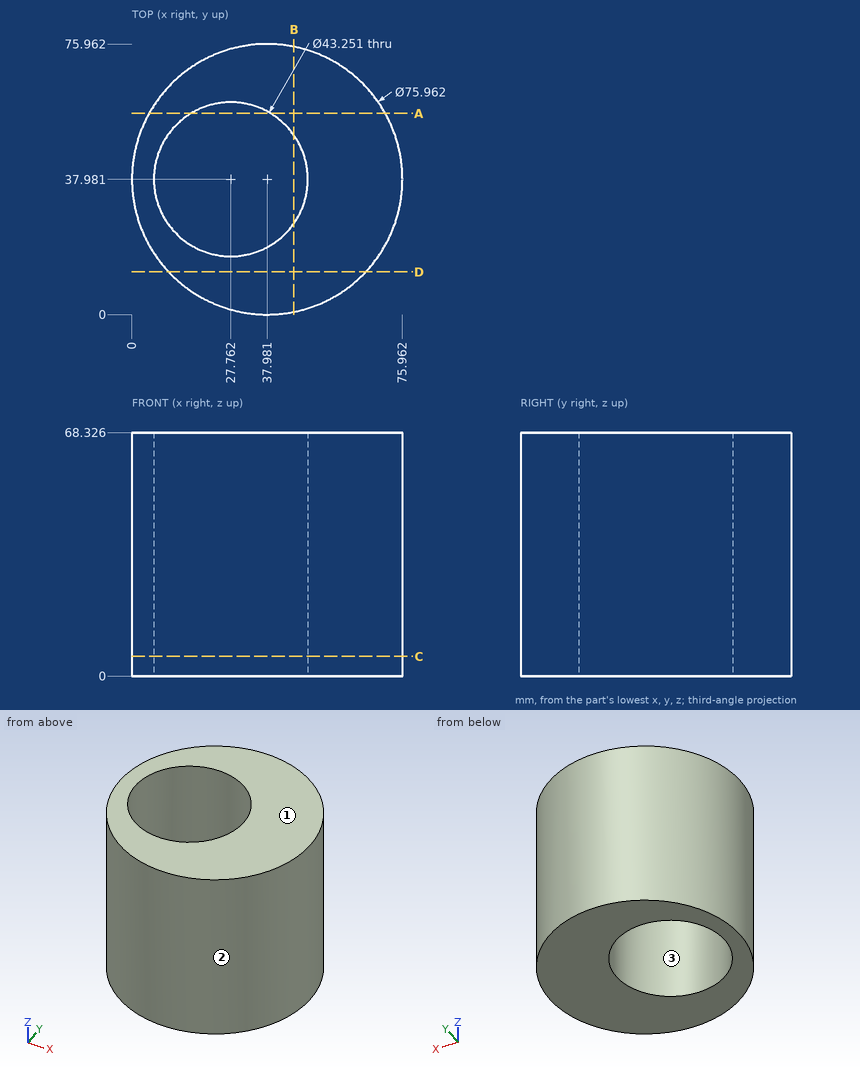
Drawing for the job (mm, zero at the part's lowest x, y, z). Round coordinates to 2 decimals unless told otherwise and drop trailing zeros. Write each loop counter-clockwise with the first axis right and the second up, starting at its lowest first coordinate (ties: lowest second). Pieces come first, ordered by that corner, then holes. Notation, with made-up numbers: (80.5, 26) - (98.5, 26) arc R18 cw to (98.5, 43) - close; hole circle Ø5 at (86, 61). An arc over 180 degrees is marked (long way). Return JSON: item names as keys, results as strings. Group by question number.
Item 1: Band-saw the part on D-D on y = 12. List the corners of the cut face in (x, z) (1 decimal), plus the area to 3 significant figures.
Item 2: Mould opens along X. For the marked faces 1, 2 and 3 say: +X half, -X half, draft (parallel to the pull), parting line (faces both ways), or undercut.
Item 3: Flat gauge pins, fed straight in: pin 1 Ø4 at (y, z) = (21.5, 9.5) entering from -X; pin 2 Ø5 at (y, z) = (30.5, 16.5) entering from -X; pin 3 Ø5 at (x, z) = (67, 17) entering from -Y. Where does each tip first touch, or does it go through?
Item 4: Band-saw the part on A-A on y = 56.5. List the corners of the cut face in (x, z).
Item 5: Probe probe 1 along Y at (x, z) = (29, 23) (1 decimal); probe 2 along Y at (x, z) = (22.5, 15.5) (1 decimal); probe 3 along X at (y, z) = (19, 9) (1 decimal). List the from-to ranges inside material, lowest first.
Item 6: Band-saw the part on B-B on x = 45.5. List the corners of the cut face in (y, z).
Item 7: Band-saw the part on C-C on z = 5.5. List the corners of the cut face in (x, y) (1 decimal).
Resolved:
{
 "1": {"outline": "(10.3, 0) - (65.7, 0) - (65.7, 68.3) - (10.3, 68.3) - close", "area": "3,790 mm²"},
 "2": {"face 1": "draft", "face 2": "parting line", "face 3": "undercut"},
 "3": {"pin 1": "stops at x = 2.87", "pin 2": "stops at x = 0.33", "pin 3": "stops at y = 10.79"},
 "4": {"outline": "(4.82, 0) - (16.59, 0) - (16.59, 68.33) - (4.82, 68.33) - close; (38.93, 0) - (71.14, 0) - (71.14, 68.33) - (38.93, 68.33) - close"},
 "5": {"probe 1": "y = 1.1 to 16.4, 59.6 to 74.9", "probe 2": "y = 3.3 to 17, 59 to 72.7", "probe 3": "x = 5.1 to 17.4, 38.1 to 70.9"},
 "6": {"outline": "(0.75, 0) - (25.61, 0) - (25.61, 68.33) - (0.75, 68.33) - close; (50.35, 0) - (75.21, 0) - (75.21, 68.33) - (50.35, 68.33) - close"},
 "7": {"outline": "circle Ø76 at (38, 38); hole circle Ø43.3 at (27.8, 38)"}
}
